from build123d import *

# Parameters (mm, degrees)
SKETCH1_R           = 8.75
BOSS_EXTRUDE1_DEPTH = 1
SKETCH2_R           = 7.9375
BOSS_EXTRUDE2_DEPTH = 3.973
SKETCH3_R           = 3.175
CUT_EXTRUDE1_DEPTH  = 5.973


with BuildPart() as part:
    # Sketch1 → Boss-Extrude1 (new body)
    with BuildSketch(Plane(origin=(0, 0, 0), x_dir=(1, 0, 0), z_dir=(0, 1, 0))):
        Circle(SKETCH1_R)
    extrude(amount=BOSS_EXTRUDE1_DEPTH)

    # Sketch2 → Boss-Extrude2 (add)
    with BuildSketch(Plane(origin=(0, 1, 0), x_dir=(1, 0, 0), z_dir=(0, 1, 0))):
        Circle(SKETCH2_R)
    extrude(amount=BOSS_EXTRUDE2_DEPTH)

    # Sketch3 → Cut-Extrude1 (cut, through all)
    with BuildSketch(Plane(origin=(0, 4.973, 0), x_dir=(1, 0, 0), z_dir=(0, 1, 0))):
        Circle(SKETCH3_R)
    extrude(amount=-CUT_EXTRUDE1_DEPTH, mode=Mode.SUBTRACT)


solid = part.part
CAD build for the part. Positions are in the model's coordinates, mm. Round coordinates to 2 decimals unless told otherwise and drop trailing zeros. Write each loop counter-clockwise with the first axis right and the second up, starting at its lowest first coordinate (ties: lowest second). Pieces come first, ordered by that corner, then holes.
(1) Slice it at D-D, the plane x = -7.5. Write the cut outline in (y, z), and give its area (3 significant figures).
(2) Drop a flat-ended pin along its axis: P1, Ø2, axis at x = -2.5, y = 4, coming from the +Z side. Give the stop position or say it passes through.
(3) Probe line 1 along Z through (x, y) = (0, 3.8) (1 decimal); line 2 along Y through (x, z) = (-8, 1.25). List the from-to ranges inside material, lowest first.
(4) Mould opens along Z. For faces 1 (the face through (-0.69, 2.52, 3.1)), 2 (the face through (-1.72, 2.96, 7.75)), 3 (the face through (2, 1, 8)) say: pulls with the +Z half, pulls with the -Z half, needs draft (parallel to the pull), parting line crosses it, or undercut.
From the geometry:
1. outline: (0, -4.51) - (1, -4.51) - (1, -2.6) - (4.97, -2.6) - (4.97, 2.6) - (1, 2.6) - (1, 4.51) - (0, 4.51) - close
1. area: 29.7 mm2
2. P1: stops at z = 7.79
3. line 1: z = -7.9 to -3.2, 3.2 to 7.9
3. line 2: y = 0 to 1
4. face 1: undercut
4. face 2: parting line crosses it
4. face 3: needs draft
